Verification items for the finished model (mm, model axes). A direction names the side the tool comes from. Coordinates: 2 decimals unless noted, no trailing zeros. Order: outer loops, then holes, each group sorted by start corner. A loop starts at its lowest first (then second) coordinate and runs counter-clockwise, first axis right, second up. Notation, with made-up numbers: M 62.25,29 L 86.25,29 A12 cw 86.25,48 Z; hole C 6.25,64 d10. An arc over 180 degrees is marked long. Answer as a JSON object with one key per item and string values. Group by question number.
(1) Access from +Z, -Z, +X, -X, +Y, -Y to the whole of each face (thin tool, end or side, straight path). Record for faces 5 (the face through (-130, 60, 0)), 6 (the face through (-460, 176, -8)), 7 (the face through (-247, 177, 10)), 8 (the face through (-480, 115, -8)).
(2) Cross-section at A-A (x = -130). Enter the section's corners in (y, z).
(3) Material ranges on line 1 (Y direction, x = -50, z = 4.25); line 2 (Z direction, x = -184.5, y = 81); line 3 (Z direction, x = -334.5, y = 10), recorded low to high.
(4) Cross-section at C-C (x = -254.5). Enter the section's corners in (y, z).
(5) Cross-section at B-B (y = 289.5). Enter the section's corners in (x, z), plus the area to 3 significant figures.
(6) Gauge pin test, flat ends, axial feed: pin 1 Ø1 at (x, z) = (-291.5, -103) entering from +Y; pin 2 Ø6 at (x, y) = (-416, 9.5) entering from +Z; pin 3 Ø1.5 at (x, z) = (-204.5, -5) entering from +Y; pin 4 Ø12 at (y, z) = (-8.5, -93.5) entering from -X. Record the tip position at first contact, or that the pin passes through.
(7) Cross-section at D-D (y = 9.5). Enter the section's corners in (x, z), plus the area to 3 significant figures.
(8) Mould release check, pull along X, two halves, no side actions. Record for faces 1 (the face through (-192.517, 299.231, 5.07)), 2 (the face through (-480, 235, -8)), 3 (the face through (-425, -8, 15)), 4 (the face through (-7.518, 342.871, 4.93)): released by +X, released by -X, zero draft, split by the parting line, or undercut.
from build123d import *

# Parameters (mm, degrees)
BOSS_EXTRUDE1_DEPTH      = 10
SKETCH2_W                = 30
SKETCH2_H                = 10
SKETCH6_W                = 15
SKETCH6_H                = 120
BOSS_EXTRUDE2_DEPTH      = 40
SKETCH7_W                = 300
SKETCH7_H                = 30
BOSS_EXTRUDE3_DEPTH      = 10
BOSS_EXTRUDE3_DEPTH_BACK = 15
SKETCH10_W               = 400
SKETCH10_H               = 300
SKETCH11_R               = 17.5
CUT_EXTRUDE1_DEPTH       = 10
LPATTERN1_COUNT          = 3
LPATTERN1_PITCH          = 80
LPATTERN1_COUNT_DIR2     = 4
LPATTERN1_PITCH_DIR2     = 80
MIRROR1_COPY_1_SKETCH_R  = 17.5
MIRROR1_COPY_1_DEPTH     = 10
MIRROR1_COPY_2_SKETCH_R  = 17.5
MIRROR1_COPY_2_DEPTH     = 10
MIRROR1_COPY_3_SKETCH_R  = 17.5
MIRROR1_COPY_3_DEPTH     = 10
MIRROR1_COPY_4_SKETCH_R  = 17.5
MIRROR1_COPY_4_DEPTH     = 10
MIRROR1_COPY_5_SKETCH_R  = 17.5
MIRROR1_COPY_5_DEPTH     = 10
MIRROR1_COPY_6_SKETCH_R  = 17.5
MIRROR1_COPY_6_DEPTH     = 10
MIRROR1_COPY_7_SKETCH_R  = 17.5
MIRROR1_COPY_7_DEPTH     = 10
MIRROR1_COPY_8_SKETCH_R  = 17.5
MIRROR1_COPY_8_DEPTH     = 10
MIRROR1_COPY_9_SKETCH_R  = 17.5
MIRROR1_COPY_9_DEPTH     = 10
MIRROR1_COPY_10_SKETCH_R = 17.5
MIRROR1_COPY_10_DEPTH    = 10
MIRROR1_COPY_11_SKETCH_R = 17.5
MIRROR1_COPY_11_DEPTH    = 10


with BuildPart() as part:
    # Sketch1 → Boss-Extrude1 (new body)
    with BuildSketch(Plane.XY):
        with BuildLine():
            Line((-475, 350), (-25, 350))
            ThreePointArc((-25, 350), (-7.32233047, 342.67766953), (0, 325))
            Line((0, 325), (0, 25))
            ThreePointArc((0, 25), (-7.32233047, 7.32233047), (-25, 0))
            Line((-25, 0), (-475, 0))
            ThreePointArc((-475, 0), (-492.67766953, 7.32233047), (-500, 25))
            Line((-500, 25), (-500, 325))
            ThreePointArc((-500, 325), (-492.67766953, 342.67766953), (-475, 350))
        make_face()
    extrude(amount=BOSS_EXTRUDE1_DEPTH)

    # Sweep1: sweep along a path in Sketch3
    with BuildLine(Plane.ZY.offset(410)) as sweep1_path:
        ThreePointArc((5, 0), (15, -10), (25, 0))
    # Sketch2 → Sweep1 (sweep)
    with BuildSketch(Plane.XZ):
        with Locations((-410, 5)):
            Rectangle(SKETCH2_W, SKETCH2_H)
    sweep1 = sweep(path=sweep1_path.line)

    # Sketch6 → Boss-Extrude2 (add)
    with BuildSketch(Plane.ZY.offset(500)):
        with Locations((-7.5, 175)):
            Rectangle(SKETCH6_W, SKETCH6_H)
    boss_extrude2 = extrude(amount=-BOSS_EXTRUDE2_DEPTH)

    # Sweep2: sweep along a path in Sketch8
    with BuildLine(Plane.ZY.offset(250)) as sweep2_path:
        Line((0, 45.401266602), (-135.946168055, -17.991472659))
    # Sketch7 → Sweep2 (sweep)
    with BuildSketch(Plane(origin=(0, 0, 0), x_dir=(-1, 0, 0), z_dir=(0, 0, -1))):
        with Locations((250, 60)):
            Rectangle(SKETCH7_W, SKETCH7_H)
    sweep(path=sweep2_path.line)

    # Sketch10 → Boss-Extrude3 (add, two sides: drawn at the far end of the back side and taken through both)
    with BuildSketch(Plane(origin=(-400, -18.392739261, -135.946168055), x_dir=(1, 0, 0), z_dir=(0, 0, 1)).offset(-BOSS_EXTRUDE3_DEPTH_BACK)):
        with Locations((150, 100)):
            Rectangle(SKETCH10_W, SKETCH10_H)
    extrude(amount=BOSS_EXTRUDE3_DEPTH + BOSS_EXTRUDE3_DEPTH_BACK)

    # Sketch11 → Cut-Extrude1 (cut)
    with BuildSketch(Plane.XY.offset(10)):
        with Locations((-450, 300)):
            Circle(SKETCH11_R)
    cut_extrude1 = extrude(amount=-CUT_EXTRUDE1_DEPTH, mode=Mode.SUBTRACT)

    # LPattern1: Cut-Extrude1 3 × 4
    with Locations(*[(i * LPATTERN1_PITCH, -j * LPATTERN1_PITCH_DIR2, 0) for i in range(LPATTERN1_COUNT) for j in range(LPATTERN1_COUNT_DIR2) if (i, j) != (0, 0)]):
        add(cut_extrude1, mode=Mode.SUBTRACT)

    # Mirror1: Sweep1, Boss-Extrude2, Cut-Extrude1 across plane
    add(sweep1.mirror(Plane.ZY.offset(250)))
    add(boss_extrude2.mirror(Plane.ZY.offset(250)))
    add(cut_extrude1.mirror(Plane.ZY.offset(250)), mode=Mode.SUBTRACT)

    # Mirror1 copy 1 sketch → Mirror1 copy 1 (cut)
    with BuildSketch(Plane(origin=(-500, -80, 10), x_dir=(-1, 0, 0), z_dir=(0, 0, 1))):
        with Locations((-450, -300)):
            Circle(MIRROR1_COPY_1_SKETCH_R)
    extrude(amount=-MIRROR1_COPY_1_DEPTH, mode=Mode.SUBTRACT)

    # Mirror1 copy 2 sketch → Mirror1 copy 2 (cut)
    with BuildSketch(Plane(origin=(-500, -160, 10), x_dir=(-1, 0, 0), z_dir=(0, 0, 1))):
        with Locations((-450, -300)):
            Circle(MIRROR1_COPY_2_SKETCH_R)
    extrude(amount=-MIRROR1_COPY_2_DEPTH, mode=Mode.SUBTRACT)

    # Mirror1 copy 3 sketch → Mirror1 copy 3 (cut)
    with BuildSketch(Plane(origin=(-500, -240, 10), x_dir=(-1, 0, 0), z_dir=(0, 0, 1))):
        with Locations((-450, -300)):
            Circle(MIRROR1_COPY_3_SKETCH_R)
    extrude(amount=-MIRROR1_COPY_3_DEPTH, mode=Mode.SUBTRACT)

    # Mirror1 copy 4 sketch → Mirror1 copy 4 (cut)
    with BuildSketch(Plane(origin=(-580, 0, 10), x_dir=(-1, 0, 0), z_dir=(0, 0, 1))):
        with Locations((-450, -300)):
            Circle(MIRROR1_COPY_4_SKETCH_R)
    extrude(amount=-MIRROR1_COPY_4_DEPTH, mode=Mode.SUBTRACT)

    # Mirror1 copy 5 sketch → Mirror1 copy 5 (cut)
    with BuildSketch(Plane(origin=(-580, -80, 10), x_dir=(-1, 0, 0), z_dir=(0, 0, 1))):
        with Locations((-450, -300)):
            Circle(MIRROR1_COPY_5_SKETCH_R)
    extrude(amount=-MIRROR1_COPY_5_DEPTH, mode=Mode.SUBTRACT)

    # Mirror1 copy 6 sketch → Mirror1 copy 6 (cut)
    with BuildSketch(Plane(origin=(-580, -160, 10), x_dir=(-1, 0, 0), z_dir=(0, 0, 1))):
        with Locations((-450, -300)):
            Circle(MIRROR1_COPY_6_SKETCH_R)
    extrude(amount=-MIRROR1_COPY_6_DEPTH, mode=Mode.SUBTRACT)

    # Mirror1 copy 7 sketch → Mirror1 copy 7 (cut)
    with BuildSketch(Plane(origin=(-580, -240, 10), x_dir=(-1, 0, 0), z_dir=(0, 0, 1))):
        with Locations((-450, -300)):
            Circle(MIRROR1_COPY_7_SKETCH_R)
    extrude(amount=-MIRROR1_COPY_7_DEPTH, mode=Mode.SUBTRACT)

    # Mirror1 copy 8 sketch → Mirror1 copy 8 (cut)
    with BuildSketch(Plane(origin=(-660, 0, 10), x_dir=(-1, 0, 0), z_dir=(0, 0, 1))):
        with Locations((-450, -300)):
            Circle(MIRROR1_COPY_8_SKETCH_R)
    extrude(amount=-MIRROR1_COPY_8_DEPTH, mode=Mode.SUBTRACT)

    # Mirror1 copy 9 sketch → Mirror1 copy 9 (cut)
    with BuildSketch(Plane(origin=(-660, -80, 10), x_dir=(-1, 0, 0), z_dir=(0, 0, 1))):
        with Locations((-450, -300)):
            Circle(MIRROR1_COPY_9_SKETCH_R)
    extrude(amount=-MIRROR1_COPY_9_DEPTH, mode=Mode.SUBTRACT)

    # Mirror1 copy 10 sketch → Mirror1 copy 10 (cut)
    with BuildSketch(Plane(origin=(-660, -160, 10), x_dir=(-1, 0, 0), z_dir=(0, 0, 1))):
        with Locations((-450, -300)):
            Circle(MIRROR1_COPY_10_SKETCH_R)
    extrude(amount=-MIRROR1_COPY_10_DEPTH, mode=Mode.SUBTRACT)

    # Mirror1 copy 11 sketch → Mirror1 copy 11 (cut)
    with BuildSketch(Plane(origin=(-660, -240, 10), x_dir=(-1, 0, 0), z_dir=(0, 0, 1))):
        with Locations((-450, -300)):
            Circle(MIRROR1_COPY_11_SKETCH_R)
    extrude(amount=-MIRROR1_COPY_11_DEPTH, mode=Mode.SUBTRACT)


solid = part.part
Taken from the geometry:
{
 "1": {"face 5": "+Z", "face 6": "-Z, +Y, -Y", "face 7": "+Z, +X, -X, +Y", "face 8": "-Z, +X, -X, -Y"},
 "2": {"outline": "M -68.39,-150.95 L 231.61,-150.95 L 231.61,-125.95 L 16.27,-125.95 L 75,0 L 45,0 L -13.73,-125.95 L -68.39,-125.95 Z; M 0,0 L 42.5,0 L 42.5,10 L 0,10 Z; M 77.5,0 L 122.5,0 L 122.5,10 L 77.5,10 Z; M 157.5,0 L 202.5,0 L 202.5,10 L 157.5,10 Z; M 237.5,0 L 282.5,0 L 282.5,10 L 237.5,10 Z; M 317.5,0 L 350,0 L 350,10 L 317.5,10 Z"},
 "3": {"line 1": "y = 0 to 42.5, 77.5 to 122.5, 157.5 to 202.5, 237.5 to 282.5, 317.5 to 350", "line 2": "z = -150.95 to -125.95, 0 to 10", "line 3": "z = -150.95 to -75.06, 0 to 10"},
 "4": {"outline": "M -68.39,-150.95 L 231.61,-150.95 L 231.61,-125.95 L 16.27,-125.95 L 75,0 L 350,0 L 350,10 L 0,10 L 0,0 L 45,0 L -13.73,-125.95 L -68.39,-125.95 Z"},
 "5": {"outline": "M -500,0 L -464,0 L -464,10 L -500,10 Z; M -436,0 L -384,0 L -384,10 L -436,10 Z; M -356,0 L -304,0 L -304,10 L -356,10 Z; M -276,0 L -224,0 L -224,10 L -276,10 Z; M -196,0 L -144,0 L -144,10 L -196,10 Z; M -116,0 L -64,0 L -64,10 L -116,10 Z; M -36,0 L 0,0 L 0,10 L -36,10 Z", "area": "3,320 mm²"},
 "6": {"pin 1": "stops at y = 27.2", "pin 2": "stops at z = 10", "pin 3": "stops at y = 73.02", "pin 4": "passes through"},
 "7": {"outline": "M -494.62,0 L -5.38,0 L -5.38,10 L -494.62,10 Z; M -450,-150.95 L -50,-150.95 L -50,-125.95 L -100,-125.95 L -100,-76.13 L -400,-76.13 L -400,-125.95 L -450,-125.95 Z", "area": "29,800 mm²"},
 "8": {"face 1": "undercut", "face 2": "zero draft", "face 3": "released by -X", "face 4": "released by +X"}
}
